Design review of the part built by this model. Coordinates are the model's own, in mm. A direction names the side the tool comes from. Round coordinates to 2 decimals unless told otherwise and drop trailing zeros. Loops run counter-clockwise (first coordinate to the right, second up) from the corner with the lowest first, then second, coordinate; pieces in that order, holes last. Notation, with made-up numbers: (-22, 25.25) - (-18, 25.25) arc R33 cw to (-18, 64.25) - close; hole circle Ø7 at (20, 45). An arc over 180 degrees is marked (long way). Return JSON: item names as keys, results as strings. Group by question number.
from build123d import *

# Parameters (mm, degrees)
F1_DEPTH    = 15.25
F2_T1_DEPTH = 107.2974570989
F3_W        = 3
F3_H        = 4
F4_ANGLE    = 180


# Not quite as in the source:
# - a fillet or chamfer that OpenCascade refuses, or shapes differently, is made with other operations: its cross-section is extruded or revolved along the edge and cut away or added


with BuildPart() as f1:
    # F0 (on Right) → F1 (new body)
    with BuildSketch(Plane.YZ):
        with BuildLine():
            Line((27.3567325823, 33.1807983013), (27.3567325823, 43.1807983013))
            ThreePointArc((27.3567325823, 43.1807983013), (22.8348355324, 42.1000161521), (19.2903756049, 39.0912877154))
            Line((19.2903756049, 39.0912877154), (27.3567325823, 33.1807983013))
        make_face()
        with BuildLine():
            Line((27.3567325823, 23.1807983013), (27.3567325823, 33.1807983013))
            Line((27.3567325823, 33.1807983013), (21.4462431681, 25.1144413239))
            ThreePointArc((21.4462431681, 25.1144413239), (24.2473572248, 23.6764948083), (27.3567325823, 23.1807983013))
        make_face()
        with BuildLine():
            Line((21.4462431681, 25.1144413239), (27.3567325823, 33.1807983013))
            Line((27.3567325823, 33.1807983013), (19.2903756049, 39.0912877154))
            ThreePointArc((19.2903756049, 39.0912877154), (17.4736097193, 31.656369728), (21.4462431681, 25.1144413239))
        make_face()
        with BuildLine():
            ThreePointArc((21.4462431681, 25.1144413239), (17.4736097193, 31.656369728), (19.2903756049, 39.0912877154))
            Line((19.2903756049, 39.0912877154), (-5.7096243951, 4.9724677154))
            ThreePointArc((-5.7096243951, 4.9724677154), (0.832304009, 8.9451011642), (8.2672219964, 7.1283352786))
            Line((8.2672219964, 7.1283352786), (21.4462431681, 25.1144413239))
        make_face()
        with BuildLine():
            ThreePointArc((-5.7096243951, 4.9724677154), (-7.1475709107, 2.1713536587), (-7.6432674177, -0.9380216987))
            Line((-7.6432674177, -0.9380216987), (2.3567325823, -0.9380216987))
            Line((2.3567325823, -0.9380216987), (-5.7096243951, 4.9724677154))
        make_face()
        with BuildLine():
            Line((27.3567325823, -0.9380216987), (27.3567325823, 23.1807983013))
            ThreePointArc((27.3567325823, 23.1807983013), (24.2473572248, 23.6764948083), (21.4462431681, 25.1144413239))
            Line((21.4462431681, 25.1144413239), (8.2672219964, 7.1283352786))
            ThreePointArc((8.2672219964, 7.1283352786), (11.2759504331, 3.5838753511), (12.3567325823, -0.9380216987))
            Line((12.3567325823, -0.9380216987), (27.3567325823, -0.9380216987))
        make_face()
        with BuildLine():
            ThreePointArc((8.2672219964, 7.1283352786), (0.832304009, 8.9451011642), (-5.7096243951, 4.9724677154))
            Line((-5.7096243951, 4.9724677154), (2.3567325823, -0.9380216987))
            Line((2.3567325823, -0.9380216987), (8.2672219964, 7.1283352786))
        make_face()
        with BuildLine():
            Line((8.2672219964, 7.1283352786), (2.3567325823, -0.9380216987))
            Line((2.3567325823, -0.9380216987), (12.3567325823, -0.9380216987))
            ThreePointArc((12.3567325823, -0.9380216987), (11.2759504331, 3.5838753511), (8.2672219964, 7.1283352786))
        make_face()
    extrude(amount=F1_DEPTH)

    # F2: fillet of radius 10 on 1 edges, made by hand

    # F2_s2 → F2_t1 (cut)
    with BuildSketch(Plane.YZ.offset(-46.0237285495)):
        with BuildLine():
            ThreePointArc((1.6177099031, 14.9724677154), (0.7648490296, 4.5400812514), (9.6840668804, -0.9380216987))
            Line((9.6840668804, -0.9380216987), (9.6840668804, -1.9380216987))
            Line((9.6840668804, -1.9380216987), (-7.6432674177, -1.9380216987))
            Line((-7.6432674177, -1.9380216987), (-8.6432674177, -0.9380216987))
            ThreePointArc((-8.6432674177, -0.9380216987), (-6.5162600928, 5.5635166568), (0.8110742054, 15.5635166568))
            Line((0.8110742054, 15.5635166568), (1.6177099031, 14.9724677154))
        make_face()
    extrude(amount=F2_T1_DEPTH, mode=Mode.SUBTRACT)

    # F3 (on face) → F4 (revolve)
    with BuildSketch(Plane.YZ.offset(15.25)):
        with Locations((28.8567325823, 4.5619783013)):
            Rectangle(F3_W, F3_H)
        Polygon((33.3567325823, 6.5619783013), (30.3567325823, 6.5619783013), (30.3567325823, 2.5619783013), (30.3567325823, 2.0619783013), (33.3567325823, 2.0619783013), align=None)
    revolve(axis=Axis((15.25, 28.8567325823, 6.5619783013), (0, 1, 0)), revolution_arc=F4_ANGLE)


solid = f1.part
Q1. Tool access review of faces 1 (the cylindrical face through (10.75, 31.88, 6.46)), 2 (the flat face through (15.25, 16, 17)): name each direction out of +Z, -Z, +X, -X, +Y, -Y from which nothing blocks a thin tool from reaching the whole face with its end or side.
Q2. Add section B-B, the plane z = 9.5. State the section outline as (x, y) points.
Q3. Insertion check: pin 1 Ø1 at (x, y) = (8.5, 14) entering from +Z; pin 2 Ø5 at (y, z) = (12.5, 36.5) entering from -X; pin 3 Ø8 at (x, z) = (6, 23) entering from +Y; pin 4 Ø1.5 at (x, y) = (8, 9.5) entering from -Z. Each pin has a flat end and moves straight along its axis. Give the tip position at first contact, or say it passes through.
Q4. Add section A-A, the plane x = 6.5. State the section outline as (y, z) points.
Q5. For line 1 (Z direction, x = 12.25, y = 27); line 2 (Z direction, x = 2, y = 2); line 3 (Y direction, x = 1.25, z = 23), list the stretches that pass through material, from the lowest coordinate up.
Q6. Add section D-D, the plane x = 12. State the section outline as (y, z) points, plus the area to 3 significant figures.
Q7. Add section C-C, the plane y = 28.5. State the section outline as (x, z) points.
Q8. Draft analysis for pull direction Y (two halves, no side actions). For faces 3 (the cylindrical face through (11.25, 28.88, 6.47)), 4 (the flat face through (0, 16, 17)), 5 (the flat face through (11, 30.357, 6)), 6 (the flat face through (13, 33.357, 7)), state which applies: pulls with the +Y half, pulls with the -Y half, needs draft (parallel to the pull), parting line crosses it, or undercut.
Evaluation:
{
 "1": {"face 1": "-X, +Y", "face 2": "+Z, -Z, +X, +Y, -Y"},
 "2": {"outline": "(0, -0.31) - (15.25, -0.31) - (15.25, 33.36) - (11.84, 33.36) - (11.84, 30.36) - (12.54, 30.36) - (12.54, 27.36) - (0, 27.36) - close"},
 "3": {"pin 1": "z = 32.55", "pin 2": "through", "pin 3": "y = 27.36", "pin 4": "z = -0.94"},
 "4": {"outline": "(1.62, 14.97) arc R10 ccw to (9.68, -0.94) - (27.36, -0.94) - (27.36, 43.18) arc R10 ccw to (19.29, 39.09) - close"},
 "5": {"line 1": "-0.94 to 43.17", "line 2": "2.66 to 15.49", "line 3": "7.5 to 27.36"},
 "6": {"outline": "(1.62, 14.97) arc R10 ccw to (9.68, -0.94) - (27.36, -0.94) - (27.36, 4.23) - (30.36, 4.23) - (30.36, 3.45) - (33.36, 3.45) - (33.36, 9.67) - (30.36, 9.67) - (30.36, 8.89) - (27.36, 8.89) - (27.36, 43.18) arc R10 ccw to (19.29, 39.09) - close", "area": "879 mm²"},
 "7": {"outline": "(15.25, 2.56) - (15.25, 10.56) arc R4 ccw to start"},
 "8": {"face 3": "undercut", "face 4": "needs draft", "face 5": "undercut", "face 6": "pulls with the +Y half"}
}
